Can you work these out from the model? Positions are in its coordinate system, mm. A direction names the side the tool comes from. Coordinates: 2 decimals unless noted, no trailing zeros. Loops run counter-clockwise (first coordinate to the right, second up) from the corner with the lowest first, then second, coordinate; pieces in that order, holes last.
```python
from build123d import *

# Parameters (mm, degrees)
F1_DEPTH = 38.1
F2_R     = 1.524
F3_R     = 1.5875
F3_R_2   = 2.54
F4_DEPTH = 2.54
F6_DEPTH = 2.54
F7_R     = 6.35


with BuildPart() as f1:
    # F0 (on Right) → F1 (new body)
    with BuildSketch(Plane.YZ):
        with BuildLine():
            Line((-54.864, 1.016), (-52.324, 1.016))
            Line((-52.324, 1.016), (-52.324, 41.402))
            ThreePointArc((-52.324, 41.402), (-51.877631, 42.479631), (-50.8, 42.926))
            Line((-50.8, 42.926), (-0.254, 42.926))
            Line((-0.254, 42.926), (-0.254, 45.466))
            Line((-0.254, 45.466), (-50.8, 45.466))
            ThreePointArc((-50.8, 45.466), (-53.673682, 44.275682), (-54.864, 41.402))
            Line((-54.864, 41.402), (-54.864, 1.016))
        make_face()
    extrude(amount=F1_DEPTH)

    # F2
    f2_edges = [f1.edges().sort_by_distance(p)[0] for p in [
        (0, -0.254, 44.196),
        (38.1, -0.254, 44.196),
    ]]
    fillet(f2_edges, radius=F2_R)

    # F3 (on face) → F4 (cut, through all)
    with BuildSketch(Plane(origin=(0, 0, 42.926), x_dir=(1, 0, 0), z_dir=(0, 0, -1))):
        with Locations((6.1595, 43.7515)):
            Circle(F3_R)
        with Locations((19.05, 39.624)):
            Circle(F3_R_2)
        with Locations((31.9405, 43.7515)):
            Circle(F3_R)
        with Locations((19.05, 7.874)):
            Circle(F3_R_2)
    extrude(amount=-F4_DEPTH, mode=Mode.SUBTRACT)

    # F5 (on face) → F6 (cut, through all)
    with BuildSketch(Plane.XZ.offset(54.864)):
        with BuildLine():
            ThreePointArc((13.97, 7.874), (14.044395, 7.694395), (14.224, 7.62))
            Line((14.224, 7.62), (23.876, 7.62))
            ThreePointArc((23.876, 7.62), (24.055605, 7.694395), (24.13, 7.874))
            Line((24.13, 7.874), (24.13, 16.891))
            ThreePointArc((24.13, 16.891), (24.055605, 17.070605), (23.876, 17.145))
            Line((23.876, 17.145), (14.224, 17.145))
            ThreePointArc((14.224, 17.145), (14.044395, 17.070605), (13.97, 16.891))
            Line((13.97, 16.891), (13.97, 7.874))
        make_face()
    extrude(amount=-F6_DEPTH, mode=Mode.SUBTRACT)

    # F7
    f7_edges = [f1.edges().sort_by_distance(p)[0] for p in [
        (38.1, -53.594, 1.016),
        (0, -53.594, 1.016),
    ]]
    fillet(f7_edges, radius=F7_R)


solid = f1.part
```
(1) I want a section at A-A on x = 19.05. Write out the boundary of the cut face in (y, z) (3 decimals).
Check values:
outline: (-54.864, 1.016) - (-52.324, 1.016) - (-52.324, 7.62) - (-54.864, 7.62) - close; (-54.864, 17.145) - (-52.324, 17.145) - (-52.324, 41.402) arc R1.524 cw to (-50.8, 42.926) - (-42.164, 42.926) - (-42.164, 45.466) - (-50.8, 45.466) arc R4.064 ccw to (-54.864, 41.402) - close; (-37.084, 42.926) - (-10.414, 42.926) - (-10.414, 45.466) - (-37.084, 45.466) - close; (-5.334, 42.926) - (-0.254, 42.926) - (-0.254, 45.466) - (-5.334, 45.466) - close
(2) Which directions (+Z, -Z, +X, -X, +Y, -Y) give clear straight access to the entire face, cutting with the end or side of a thin tool? Please do faces 5 (the flat face through (19, -52.324, 21)), 6 (the cylindrical face through (36.289, -53.576, 2.926)), 7 (the flat face through (19, -54, 17.145)).
Check values:
face 5: -Z, +X, -X, +Y
face 6: -Z, +X, +Y, -Y
face 7: +Y, -Y
(3) If we mould it in two halves opening along X, with no side actions, what happens to faces 1 (the flat face through (0, -36.3, 43.4)), 2 (the cylindrical face through (31.6, -42.2, 44.2)), 3 (the cylindrical face through (17.034, -6.328, 44.178)), 4 (the cylindrical face through (18.78, -53.64, 44.31))? For each: released by +X, released by -X, zero draft, split by the parting line, or undercut.
Check values:
face 1: released by -X
face 2: undercut
face 3: undercut
face 4: zero draft
(4) I want a section at B-B on x = 25. Write out the boundary of the cut face in (y, z).
Check values:
outline: (-54.86, 1.02) - (-52.32, 1.02) - (-52.32, 41.4) arc R1.52 cw to (-50.8, 42.93) - (-0.25, 42.93) - (-0.25, 45.47) - (-50.8, 45.47) arc R4.06 ccw to (-54.86, 41.4) - close
(5) I want a section at C-C on y = -38. Write out the boundary of the cut face in (x, z).
Check values:
outline: (0, 42.93) - (17.1, 42.93) - (17.1, 45.47) - (0, 45.47) - close; (21, 42.93) - (38.1, 42.93) - (38.1, 45.47) - (21, 45.47) - close
(6) I'm going to push flat-ended pins straight in: pin 1 (6 mm diameter, centred on x = 29, z = 26.5, fed in from +Y); pin 2 (1.9 mm diameter, centred on x = 6.16, y = -43.75, fed in from -Z); pin 3 (1.3 mm diameter, centred on x = 17.5, y = -53.5, fed in from +Z); pin 4 (6 mm diameter, centred on x = 8, y = -41, fed in from -Z). Where does each tip first touch, or does it pass through?
Check values:
pin 1: stops at y = -52.32
pin 2: passes through
pin 3: stops at z = 44.91
pin 4: stops at z = 42.93
(7) If I drill on probe 1 along Y at (x, z) = (19.05, 44.55); probe 2 along Y at (x, z) = (19.05, 44.35); probe 3 along Z at (x, y) = (3, -8), over which ranges is the centre line in solid material (lowest first)?
Check values:
probe 1: y = -53.37 to -42.16, -37.08 to -10.41, -5.33 to -0.25
probe 2: y = -53.6 to -42.16, -37.08 to -10.41, -5.33 to -0.25
probe 3: z = 42.93 to 45.47
(8) I want a section at D-D on z = 30. Write out the boundary of the cut face in (x, y).
Check values:
outline: (0, -54.86) - (38.1, -54.86) - (38.1, -52.32) - (0, -52.32) - close
